Source: three-view drawing plus pictorial views. Frame: mm from the lowest corner of the part. Give positions to 0.01 mm unless a question says otherwise; leave off trailing zeros. Order: outer loops, then holes, each group sorted by start corner. A loop starts at its lowest first (then second) coordinate and runs counter-clockwise, first axis right, second up. Notation, with made-up numbers: (-27, 73) -> (6, 73) arc R15 ccw to (6, 101) -> close; hole circle Ø9 at (-7.5, -9). An arc over 180 degrees is marked (long way). Answer in a Markdown table with one row per item.
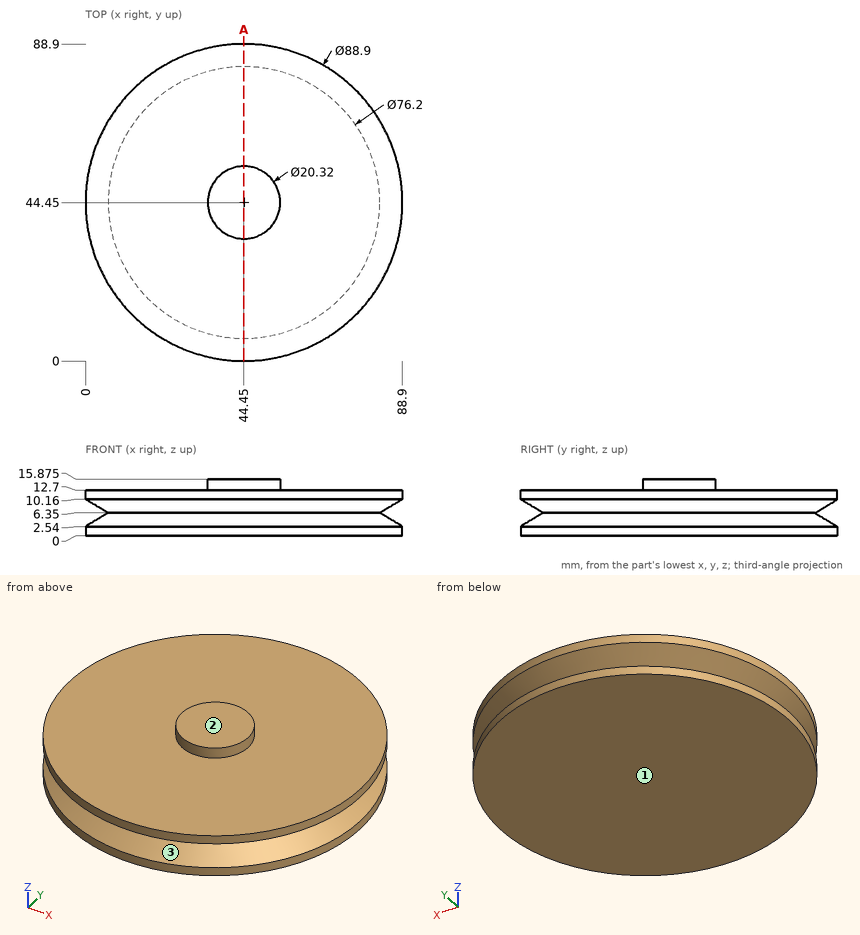
(1) Section query A-A (x = 44.45). Return the cut outline in (y, z) (3 decimals).
A:
| item | result |
|---|---|
| outline | (0, 0) -> (88.9, 0) -> (88.9, 2.54) -> (82.55, 6.35) -> (88.9, 10.16) -> (88.9, 12.7) -> (54.61, 12.7) -> (54.61, 15.875) -> (34.29, 15.875) -> (34.29, 12.7) -> (0, 12.7) -> (0, 10.16) -> (6.35, 6.35) -> (0, 2.54) -> close |
(2) First-contact query: pin 1 Ø1 at (y, z) = (61, 2.5) entering from +X; pin 2 Ø1 at (x, z) = (45, 7.5) entering from +Y; pin 3 Ø4 at (y, z) = (73.5, 5.5) entering from -X. Flat tips, straight axial feed; report the tip coordinate or a pass-through.
A:
| item | result |
|---|---|
| pin 1 | stops at x = 85.9 |
| pin 2 | stops at y = 85.3 |
| pin 3 | stops at x = 12.6 |
(3) Ray query, probe 1 along Z at (x, y) = (57, 60.5); probe 2 along Z at (x, y) = (82.5, 65); probe 3 along Y at (x, z) = (44, 13). Return the intervals inside material, ascending.
A:
| item | result |
|---|---|
| probe 1 | z = 0 to 12.7 |
| probe 2 | z = 0 to 3.26, 9.44 to 12.7 |
| probe 3 | y = 34.3 to 54.6 |
(4) Pull-direction query (Z, two-part tool) for the marked faces 1, 2 and 3; classes: +Z half, -Z half, draft (parallel to the pull), parting line (faces both ways), or undercut.
A:
| item | result |
|---|---|
| face 1 | -Z half |
| face 2 | +Z half |
| face 3 | undercut |
